```python
from build123d import *

# Parameters (mm, degrees)
SKETCH1_R           = 20
BOSS_EXTRUDE1_DEPTH = 10
SKETCH2_R           = 6.25
BOSS_EXTRUDE2_DEPTH = 152
CUT_EXTRUDE2_START  = -10
CUT_EXTRUDE2_DEPTH  = 10
CIRPATTERN1_COUNT   = 3
SKETCH8_R           = 8
CUT_EXTRUDE3_DEPTH  = 1


with BuildPart() as part:
    # Sketch1 → Boss-Extrude1 (new body)
    with BuildSketch(Plane(origin=(0, 0, 0), x_dir=(1, 0, 0), z_dir=(0, 1, 0))):
        with Locations(Location((0, 0, 0), (0, 0, 270))):
            Circle(SKETCH1_R)
    extrude(amount=-BOSS_EXTRUDE1_DEPTH)

    # Sketch2 → Boss-Extrude2 (add)
    with BuildSketch(Plane(origin=(0, 0, 0), x_dir=(1, 0, 0), z_dir=(0, 1, 0))):
        with Locations(Location((0, 0, 0), (0, 0, 270))):
            Circle(SKETCH2_R)
    extrude(amount=BOSS_EXTRUDE2_DEPTH)

    # Sketch7 → Cut-Extrude2 (cut)
    with BuildSketch(Plane(origin=(0, 152, 0), x_dir=(1, 0, 0), z_dir=(0, 1, 0)).offset(CUT_EXTRUDE2_START)):
        with BuildLine():
            Line((-1.75, 6), (1.75, 6))
            ThreePointArc((1.75, 6), (0, 6.25), (-1.75, 6))
        make_face()
    cut_extrude2 = extrude(amount=CUT_EXTRUDE2_DEPTH, mode=Mode.SUBTRACT)

    # CirPattern1: Cut-Extrude2 ×3 about axis
    cirpattern1_axis = Axis((0, 0, 0), (0, 1, 0))
    for i in range(1, CIRPATTERN1_COUNT):
        add(cut_extrude2.rotate(cirpattern1_axis, i * 360 / CIRPATTERN1_COUNT), mode=Mode.SUBTRACT)

    # Sketch8 → Cut-Extrude3 (cut)
    with BuildSketch(Plane.XZ.offset(10)):
        with Locations(Location((0, 0, 0), (0, 0, 270))):
            Circle(SKETCH8_R)
    extrude(amount=-CUT_EXTRUDE3_DEPTH, mode=Mode.SUBTRACT)


solid = part.part
```
The model under review builds one solid part; all positions refer to its coordinate system, in mm. A direction names the side the tool comes from. Coordinates: 2 decimals unless noted, no trailing zeros. Write each loop counter-clockwise with the first axis right and the second up, starting at its lowest first coordinate (ties: lowest second). Pieces come first, ordered by that corner, then holes. Notation, with made-up numbers: (3, 41) - (44, 41) arc R29 cw to (44, 64) - close; hole circle Ø8 at (-9, -3.5). An arc over 180 degrees is marked (long way). Answer in a Markdown table with one row per item. Add a question column.
Q1. Consider section D-D on x = 10. Give the boundary of the cut face in (y, z).
Q2. Clearance check with flat-ended pins moving along their axes: pin 1 (8 mm diameter, centred on y = 14.5, z = -12, fed in from -X); pin 2 (6 mm diameter, centred on x = 13.5, z = 12.5, fed in from +Y); pin 3 (17.5 mm diameter, centred on x = 4, z = -2, fed in from -Y); pin 4 (4 mm diameter, centred on x = -0.5, y = 145.5, fed in from -Z). State where each tip first meets the part, or that it passes through.
Q3. Consider section B-B on x = 0. Give the boundary of the cut face in (y, z).
Q4. Consider section A-A on z = 0. Give the boundary of the cut face in (x, y).
Q5. For faces 5 (the face through (5.21, 146.93, 2.98)), 6 (the face through (5, 0, 4)), 7 (the face through (0, -9, 0)), 8 (the face through (-19.524, -4.93, -4.336)), 9 (the face through (0, -10, 9)), list the 3-axis set-ups (+Z, -Z, +X, -X, +Y, -Y) from which the entire face can be reached by the end or side of a thin tool; tool diameter is ignored.
Q6. To check wall thickness, follow line 1 along X through (y, z) = (-9.4, 0); line 2 along Y through (x, z) = (1, -10.5); line 3 along Y through (x, z) = (-1, 6). State the ranges of each line that lie inside material, in increasing order. Write a range as from..to.
Q7. Consider section C-C on y = 81. Give the boundary of the cut face in (x, z), then the cut area to 3 significant figures.
Q8. Draft analysis for pull direction Z (two halves, no side actions). For faces 1 (the face through (0, 147, -6)), 2 (the face through (-7.81, -9.51, 1.73)), 3 (the face through (-5.184, 146.93, 3.021)), 4 (the face through (1.88, 74.94, 5.96)), state which applies: +Z half, -Z half, draft (parallel to the pull), parting line (faces both ways), or undercut.
Answers below:
| question | item | result |
|---|---|---|
| 1 | outline | (-10, -17.32) - (0, -17.32) - (0, 17.32) - (-10, 17.32) - close |
| 2 | pin 1 | through |
| 2 | pin 2 | y = 0 |
| 2 | pin 3 | y = -10 |
| 2 | pin 4 | z = -6 |
| 3 | outline | (-10, -20) - (0, -20) - (0, -6.25) - (142, -6.25) - (142, -6) - (152, -6) - (152, 6.25) - (0, 6.25) - (0, 20) - (-10, 20) - (-10, 8) - (-9, 8) - (-9, -8) - (-10, -8) - close |
| 4 | outline | (-20, -10) - (-8, -10) - (-8, -9) - (8, -9) - (8, -10) - (20, -10) - (20, 0) - (6.25, 0) - (6.25, 152) - (-6.25, 152) - (-6.25, 0) - (-20, 0) - close |
| 5 | face 5 | +Z, +X, +Y |
| 5 | face 6 | +Y |
| 5 | face 7 | -Y |
| 5 | face 8 | +Y, -Y |
| 5 | face 9 | +Z, -Z, +X, -X, -Y |
| 6 | line 1 | -20..-8, 8..20 |
| 6 | line 2 | -10..0 |
| 6 | line 3 | -9..152 |
| 7 | outline | circle Ø12.5 at (0, 0) |
| 7 | area | 123 mm² |
| 8 | face 1 | -Z half |
| 8 | face 2 | undercut |
| 8 | face 3 | +Z half |
| 8 | face 4 | parting line |
